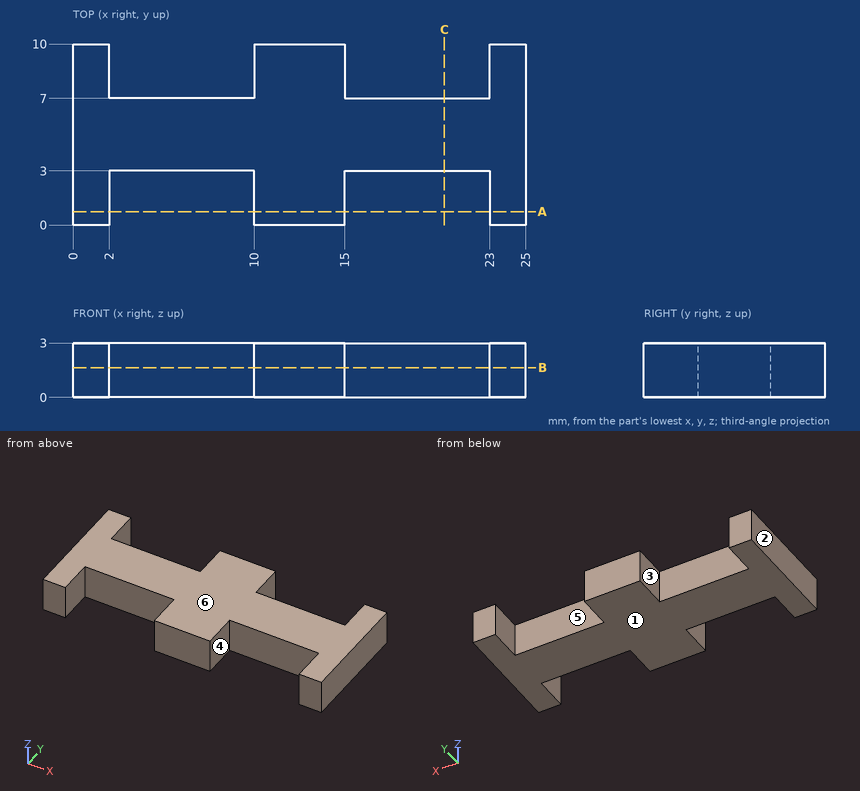
Geometry: see drawing. Coordinates: mm, zero at the bounding-box minimum. A direction names the side the tool comes from. Round coordinates to 2 decimals unless told otherwise and drop trailing zeros. Write each loop counter-clockwise with the first axis right and the second up, starting at its lowest first coordinate (ties: lowest second). Pieces come first, ordered by that corner, then holes.
Item 1: Material intervals for L1, parallel to X at y = 8.5, z = 0.3; L2, parallel to Y at x = 17.5, z = 1.3, sorted ascending.
Item 2: Set-up query: the marked faces 4, 5 and 6. Return all of +Z, -Z, +X, -X, +Y, -Y with unobstructed straight access to the full face (end or side cutting, diameter ignored); none if empty.
Item 3: Section query B-B (z = 1.65). Return loops of the section in (x, y).
Item 4: Pin query (flat end, axial travel): P1, Ø1.5, axis at x = 5.5, z = 1, coming from the -Y side; P2, Ø1.5, axis at x = 19.5, z = 1, coming from the +Y side. Return the tip coordinate at first contact, or that it passes through.
Item 5: Section query A-A (y = 0.75). Return loops of the section in (x, z).
Item 6: Mould query, pull axis X, two halves, no side actions, for the marked faces 1, 2 and 3. Classes: +X half, -X half, draft (parallel to the pull), parting line (faces both ways), or undercut.
Item 7: Section query C-C (x = 20.5). Return loops of the section in (y, z), plus the area to 3 significant figures.
Completed:
1. L1: x = 0 to 2, 10 to 15, 23 to 25
1. L2: y = 3 to 7
2. face 4: +Z, -Z, -Y
2. face 5: +Z, -Z, +Y
2. face 6: +Z, +X, -X, +Y, -Y
3. outline: (0, 0) - (2, 0) - (2, 3) - (10, 3) - (10, 0) - (15, 0) - (15, 3) - (23, 3) - (23, 0) - (25, 0) - (25, 10) - (23, 10) - (23, 7) - (15, 7) - (15, 10) - (10, 10) - (10, 7) - (2, 7) - (2, 10) - (0, 10) - close
4. P1: stops at y = 3
4. P2: stops at y = 7
5. outline: (0, 0) - (2, 0) - (2, 3) - (0, 3) - close; (10, 0) - (15, 0) - (15, 3) - (10, 3) - close; (23, 0) - (25, 0) - (25, 3) - (23, 3) - close
6. face 1: draft
6. face 2: -X half
6. face 3: undercut
7. outline: (3, 0) - (7, 0) - (7, 3) - (3, 3) - close
7. area: 12.0 mm2
